Part model, mm, in its own coordinate system. A direction names the side the tool comes from. Round coordinates to 2 decimals unless told otherwise and drop trailing zeros. Loops run counter-clockwise (first coordinate to the right, second up) from the corner with the lowest first, then second, coordinate; pieces in that order, holes last.
(1) Probe probe 1 along Y at (x, z) = (10, 1.65); probe 2 along Y at (x, z) = (44, 2.5); probe 3 along X at (y, z) = (-102, 0.4). List the from-to ranges inside material, lowest first.
(2) Mould opens along X. For faces 3 (the face through (54, 0, 1)), 4 (the face through (9.71, -101.82, 1.48)), 5 (the face through (8.38, -8.51, 1.48)), 6 (the face through (0, -58, 1)) say: +X half, -X half, draft (parallel to the pull), parting line (faces both ways), or undercut.
(3) Cut at A-A on y = -68. List the corners of the cut face in (x, z).
(4) Tool access for faces 1 (the face through (54, -44, 0)), 2 (the face through (70, -60, 1)): list every direction of +Z, -Z, +X, -X, +Y, -Y with a clear straight run to the whole face (end or side of a thin tool).
(5) Cut at C-C on z = 1.75. List the corners of the cut face in (x, y), then the cut area to 3 significant figures.
(6) Cut at B-B on x = 24. List the corners of the cut face in (y, z).
from build123d import *

# Parameters (mm, degrees)
SKETCH_1_W      = 109
SKETCH_1_H      = 114
SKETCH_1_R      = 2.2
SKETCH_1_W_2    = 56
SKETCH_1_H_2    = 26
EXTRUDE_1_DEPTH = 3
FILLET_2_R      = 2
FILLET_3_R      = 10


with BuildPart() as part:
    # 草图1 → 凸台-拉伸1 (new body)
    with BuildSketch(Plane.XY):
        with Locations((54.5, -57)):
            Rectangle(SKETCH_1_W, SKETCH_1_H)
        with Locations((99, -10)):
            Circle(SKETCH_1_R, mode=Mode.SUBTRACT)
        with Locations((99, -104)):
            Circle(SKETCH_1_R, mode=Mode.SUBTRACT)
        with Locations((10, -10)):
            Circle(SKETCH_1_R, mode=Mode.SUBTRACT)
        with Locations((10, -104)):
            Circle(SKETCH_1_R, mode=Mode.SUBTRACT)
        with Locations((42, -60)):
            Rectangle(SKETCH_1_W_2, SKETCH_1_H_2, mode=Mode.SUBTRACT)
    extrude(amount=EXTRUDE_1_DEPTH)

    # 圆角2
    fillet_2_edges = [part.edges().sort_by_distance(p)[0] for p in [
        (14, -47, 1.5),
        (14, -73, 1.5),
        (70, -73, 1.5),
        (70, -47, 1.5),
    ]]
    fillet(fillet_2_edges, radius=FILLET_2_R)

    # 圆角3
    fillet_3_edges = [part.edges().sort_by_distance(p)[0] for p in [
        (0, 0, 1.5),
        (109, 0, 1.5),
        (109, -114, 1.5),
        (0, -114, 1.5),
    ]]
    fillet(fillet_3_edges, radius=FILLET_3_R)


solid = part.part
Final values:
1. probe 1: y = -114 to -106.2, -101.8 to -12.2, -7.8 to 0
1. probe 2: y = -114 to -73, -47 to 0
1. probe 3: x = 0 to 9.08, 10.92 to 98.08, 99.92 to 109
2. face 3: draft
2. face 4: undercut
2. face 5: undercut
2. face 6: -X half
3. outline: (0, 0) - (14, 0) - (14, 3) - (0, 3) - close; (70, 0) - (109, 0) - (109, 3) - (70, 3) - close
4. face 1: -Z, +X, -X, +Y, -Y
4. face 2: +Z, -Z
5. outline: (0, -104) arc R10 ccw to (10, -114) - (99, -114) arc R10 ccw to (109, -104) - (109, -10) arc R10 ccw to (99, 0) - (10, 0) arc R10 ccw to (0, -10) - close; hole circle Ø4.4 at (10, -104); hole circle Ø4.4 at (10, -10); hole (14, -71) arc R2 ccw to (16, -73) - (68, -73) arc R2 ccw to (70, -71) - (70, -49) arc R2 ccw to (68, -47) - (16, -47) arc R2 ccw to (14, -49) - close; hole circle Ø4.4 at (99, -104); hole circle Ø4.4 at (99, -10)
5. area: 10,800 mm2
6. outline: (-114, 0) - (-73, 0) - (-73, 3) - (-114, 3) - close; (-47, 0) - (0, 0) - (0, 3) - (-47, 3) - close
